Geometry check sheet. Reference: the model listing, model coordinates, mm. Coordinates: 2 decimals unless noted, no trailing zeros. Write each loop counter-clockwise with the first axis right and the second up, starting at its lowest first coordinate (ties: lowest second). Pieces come first, ordered by that corner, then holes. Notation, with made-up numbers: (79, 20) -> (136, 20) arc R12 ccw to (136, 25) -> close; hole circle Ø3 at (-24.75, -31.75). An arc over 180 degrees is marked (long way). Answer in a Markdown table with one row per item. Add a question column.
Q1. Release check for a two-part mould opening along X. For faces 1 (the face through (0, 3, 203.2)), 2 (the face through (1.204, 3.131, -39.026)), 3 (the face through (-44.45, 3, -3)) record: pulls with the +X half, pulls with the -X half, needs draft (parallel to the pull), parting line crosses it, or undercut.
Q2. Section check B-B, the plane z = -44.45. Record the boundary of the cut face in (x, y).
Q3. Section check D-D, the plane x = -39. Record the boundary of the cut face in (y, z), and give its area (3 significant figures).
Q4. Thickness scan on line 1 (Z direction, x = 8, y = 4.75); line 2 (X direction, y = 1.5, z = -144.4); line 3 (Z direction, x = 35.5, y = 4.75). Record the ranges inside material, lowest first.
Q5. Section check A-A, the plane y = 2.25. Count the separate pieces of the cut face and the enclosed holes in it, and give its area (3 significant figures).
Q6. Section check C-C, the plane x = 37.5. Record the boundary of the cut face in (y, z).
Autodesk Inventor part; units mm, degrees
ref_plane "YZ Plane" through (0, 0, 0) normal (1, 0, 0) x (0, 1, 0)
ref_plane "XZ Plane" through (0, 0, 0) normal (0, 1, 0) x (-1, 0, 0)
ref_plane "XY Plane" through (0, 0, 0) normal (0, 0, 1) x (1, 0, 0)
sketch "Sketch1" plane through (0, 0, 0) normal (0, 1, 0) x (-1, 0, 0)
  line L0 (-44.45, -203.2) -> (44.45, -203.2)
  line L1 (44.45, -203.2) -> (44.45, 203.2)
  line L2 (44.45, 203.2) -> (-44.45, 203.2)
  line L3 (-44.45, 203.2) -> (-44.45, -203.2)
  line L4 (-44.45, -203.2) -> (44.45, 203.2) construction
  line L5 (44.45, -203.2) -> (-44.45, 203.2) construction
  line L6 (0, 203.2) -> (0, -203.2) construction
  line L7 (0, 0) -> (44.45, 0) construction
  line L8 (0, -203.2) -> (0, 203.2) construction
  line L9 (0, 152.4) -> (7.112, 152.4) construction
  line L10 (0, -152.4) -> (0, -203.2) construction
  circle A0 centre (0, -152.4) radius 4
  circle A1 centre (0, -152.4) radius 8 construction
  line L11 (0, 152.4) -> (-44.45, 152.4) construction
  line L12 (-44.45, 152.4) -> (-44.45, 88.9)
  line L13 (-44.45, 88.9) -> (0, 88.9) construction
  line L14 (0, 88.9) -> (0, 152.4) construction
  circle A2 centre (0, -144.4) radius 1.85
  circle A3 centre (-8, -152.4) radius 1.85
  circle A4 centre (0, -160.4) radius 1.85
  circle A5 centre (8, -152.4) radius 1.85
  circle A6 centre (0, 152.4) radius 4
  circle A7 centre (0, 152.4) radius 8 construction
  circle A8 centre (0, 160.4) radius 1.85
  circle A9 centre (0, 152.4) radius 8 construction
  circle A10 centre (-8, 152.4) radius 1.85
  circle A11 centre (0, 152.4) radius 8 construction
  circle A12 centre (0, 144.4) radius 1.85
  circle A13 centre (0, 152.4) radius 8 construction
  circle A14 centre (8, 152.4) radius 1.85
  line L15 (-88.9, 44.45) -> (0, 44.45) construction
  line L16 (0, 44.45) -> (0, -44.45) construction
  line L17 (0, -44.45) -> (-88.9, -44.45) construction
  line L18 (-88.9, -44.45) -> (-88.9, 44.45) construction
  line L19 (-88.9, 44.45) -> (0, -44.45) construction
  line L20 (0, 44.45) -> (-88.9, -44.45) construction
  circle A15 centre (0, 44.45) radius 5.5563
  circle A16 centre (0, -44.45) radius 5.5563
  point P0 (-44.45, 0)
  dimension "d17" = 16
  dimension "d40" = 16
  dimension "d0" = 406.4
  dimension "d1" = 88.9
  dimension "d2" = 152.4
  dimension "d16" = 8
  dimension "d24" = 44.45
  dimension "d25" = 63.5
  dimension "d34" = 3.7
  dimension "d37" = 360
  dimension "d39" = 8
  dimension "d41" = 3.7
  dimension "d44" = 360
  dimension "d63" = 88.9
  dimension "d64" = 11.1125
  dimension "d65" = 11.1125
extrude "Extrusion6" add sketch "Sketch1" along normal blind 6.35
chamfer "Chamfer6" distance 20.32 angle 45 4 edges at (-44.45, 3.175, 203.2) (44.45, 3.175, 203.2) (44.45, 3.175, -203.2) (-44.45, 3.175, -203.2)
properties part number "testPart_chassis2"
Calculated:
| question | item | result |
|---|---|---|
| 1 | face 1 | needs draft |
| 1 | face 2 | undercut |
| 1 | face 3 | pulls with the -X half |
| 2 | outline | (-44.45, 0) -> (-5.56, 0) -> (-5.56, 6.35) -> (-44.45, 6.35) -> close; (5.56, 0) -> (44.45, 0) -> (44.45, 6.35) -> (5.56, 6.35) -> close |
| 3 | outline | (0, -188.33) -> (6.35, -188.33) -> (6.35, 188.33) -> (0, 188.33) -> close |
| 3 | area | 2,390 mm² |
| 4 | line 1 | z = -203.2 to -154.25, -150.55 to 150.55, 154.25 to 203.2 |
| 4 | line 2 | x = -44.45 to -1.85, 1.85 to 44.45 |
| 4 | line 3 | z = -191.83 to 191.83 |
| 5 | separate pieces | 1 |
| 5 | enclosed holes | 12 |
| 5 | area | 34,900 mm² |
| 6 | outline | (0, -189.83) -> (6.35, -189.83) -> (6.35, 189.83) -> (0, 189.83) -> close |
